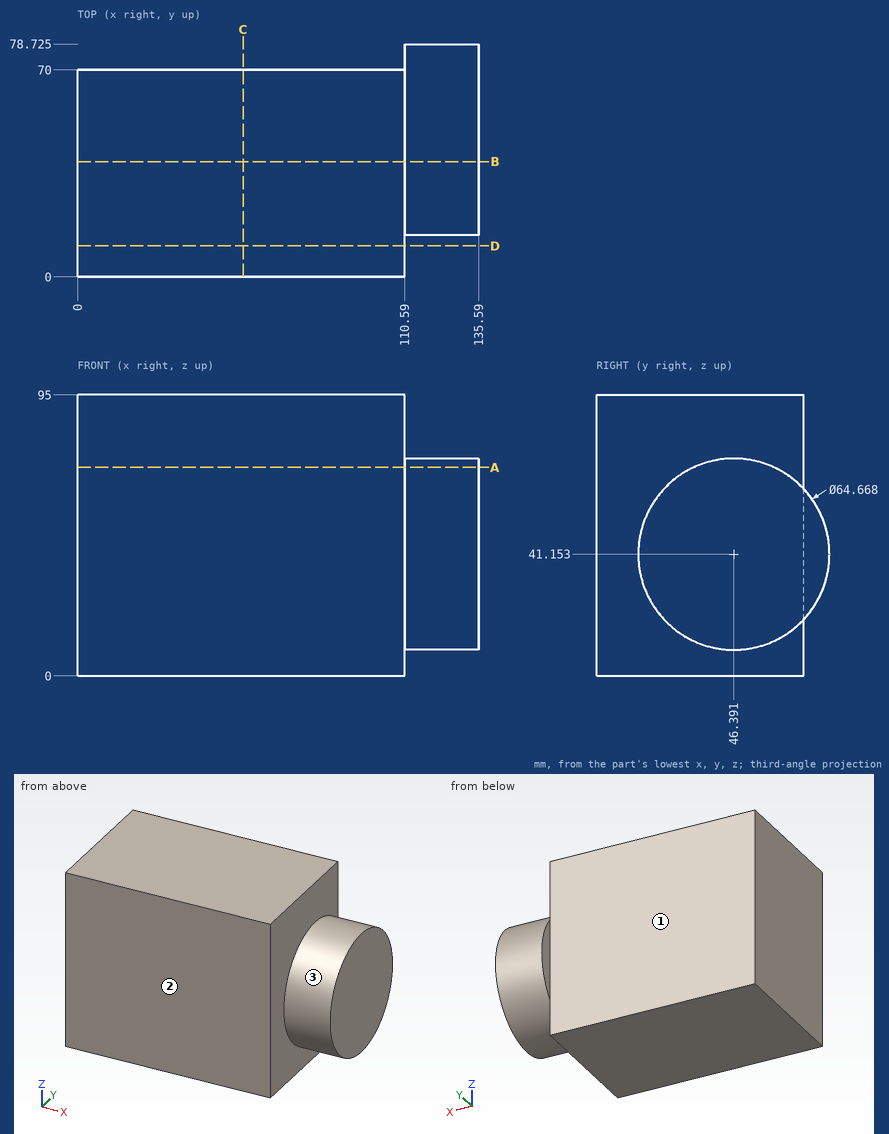
Check sheet for the drawn part. Datum: minimum x, y, z corner. Units: mm. A direction names the side the tool comes from. Give positions to 0.01 mm unless a question says otherwise; leave off trailing zeros. Write each loop counter-clockwise with the first axis right and the second up, starting at its lowest first coordinate (ties: lowest second). Pieces come first, ordered by that corner, then holes. Notation, with made-up numbers: (32.25, 22.25) - (52.25, 22.25) arc R23 cw to (52.25, 42.25) - close; hole circle Ø4 at (-11, 5.5). An arc over 180 degrees is marked (long way). Put each result on its own line as item: value.
1. Sectioned sample at A-A, the plane z = 70.5. Enter the section's corners in (x, y) (1 decimal), plus the area to 3 significant figures.
Ans:
outline: (0, 0) - (110.6, 0) - (110.6, 32.8) - (135.6, 32.8) - (135.6, 60) - (110.6, 60) - (110.6, 70) - (0, 70) - close
area: 8,420 mm²
2. Thickness scan on line 1 (X direction, y = 10, z = 19.5); line 2 (Y direction, x = 103, z = 24); line 3 (Y direction, x = 112.5, z = 39). Record the ranges inside material, lowest first.
Ans:
line 1: x = 0 to 110.59
line 2: y = 0 to 70
line 3: y = 14.13 to 78.65
3. Sectioned sample at C-C, the plane x = 56. Enter the section's corners in (y, z).
Ans:
outline: (0, 0) - (70, 0) - (70, 95) - (0, 95) - close
4. Sectioned sample at D-D, the plane y = 10.5. Enter the section's corners in (x, z).
Ans:
outline: (0, 0) - (110.59, 0) - (110.59, 95) - (0, 95) - close
5. Go/stop test with flat-tipped pins: pin 1 (6 mm diameter, centred on x = 40, z = 43.5, fed in from +Y); pin 2 (9.5 mm diameter, centred on y = 75, z = 35, fed in from -X). Record where each tip stops, or that it passes through.
Ans:
pin 1: stops at y = 70
pin 2: stops at x = 110.59
6. Sectioned sample at B-B, the plane y = 39. Enter the section's corners in (x, z) (1 decimal), plus the area to 3 significant figures.
Ans:
outline: (0, 0) - (110.6, 0) - (110.6, 9.7) - (135.6, 9.7) - (135.6, 72.6) - (110.6, 72.6) - (110.6, 95) - (0, 95) - close
area: 12,100 mm²
7. Set-up check for the marked faces 1, 2 and 3: record each of +Z, -Z, +X, -X, +Y, -Y from which the full face is reachable in a straight line by a thin tool's end or side.
Ans:
face 1: +Z, -Z, -X, +Y
face 2: +Z, -Z, +X, -X, -Y
face 3: +X
